from build123d import *

# Parameters (mm, degrees)
CROQUIS6_R              = 7
CROQUIS6_R_2            = 1.4
SALIENTE_EXTRUIR4_DEPTH = 5
REDONDEO2_R             = 3
CROQUIS7_R              = 3
CORTAR_EXTRUIR2_DEPTH   = 3


with BuildPart() as part:
    # Croquis6 → Saliente-Extruir4 (new body)
    with BuildSketch(Plane.ZY.offset(29.169607513)):
        with Locations((65.25, 31.063666838)):
            Circle(CROQUIS6_R)
        with Locations((65.25, 31.063666838)):
            Circle(CROQUIS6_R_2, mode=Mode.SUBTRACT)
    extrude(amount=SALIENTE_EXTRUIR4_DEPTH)

    # Redondeo2
    redondeo2_edges = [part.edges().sort_by_distance(p)[0] for p in [
        (-34.169607513, 31.063666838, 58.25),
    ]]
    fillet(redondeo2_edges, radius=REDONDEO2_R)

    # Croquis7 → Cortar-Extruir2 (cut)
    with BuildSketch(Plane.ZY.offset(34.169607513)):
        with Locations((65.25, 31.063666838)):
            Circle(CROQUIS7_R)
    extrude(amount=-CORTAR_EXTRUIR2_DEPTH, mode=Mode.SUBTRACT)


solid = part.part
Build history of the part. All positions in model axes, mm. A direction names the side the tool comes from. Round coordinates to 2 decimals unless told otherwise and drop trailing zeros. Write each loop counter-clockwise with the first axis right and the second up, starting at its lowest first coordinate (ties: lowest second). Pieces come first, ordered by that corner, then holes. Notation, with made-up numbers: M 89.25,5 L 106.25,5 A32 ccw 106.25,40 Z; hole C 22,89.25 d2. An arc over 180 degrees is marked long. Answer in a Markdown table with one row per item.
1. Flat gauge pins, fed straight in: P1, Ø1.8, axis at y = 30.5, z = 64, coming from the -X side; P2, Ø1, axis at x = -33.5, z = 62, coming from the -Y side; P3, Ø1.5, axis at x = -30.5, z = 63, coming from the +Y side. Where does each tip first touch, or does it go through?
Geometry check:
| item | result |
|---|---|
| P1 | x = -31.17 |
| P2 | y = 25.5 |
| P3 | y = 37.9 |
2. Saw through at C-C (x = -30.1). List the corners of the cut face in (y, z).
Geometry check:
| item | result |
|---|---|
| outline | C 31.06,65.25 d14; hole C 31.06,65.25 d2.8 |
3. Saw through at A-A (z = 65.25). List the corners of the cut face in (x, y).
Geometry check:
| item | result |
|---|---|
| outline | M -34.17,27.06 A3 ccw -31.17,24.06 L -29.17,24.06 L -29.17,29.66 L -31.17,29.66 L -31.17,28.06 L -34.17,28.06 Z; M -34.17,34.06 L -31.17,34.06 L -31.17,32.46 L -29.17,32.46 L -29.17,38.06 L -31.17,38.06 A3 ccw -34.17,35.06 Z |
4. Probe L1, parallel to Y at x = -30.65, z = 65.25; L2, parallel to Y at x = -33.5, z = 62.5; L3, parallel to Z at x = -31.85, y = 29.75. List the from-to ranges inside material, lowest first. Write a range as [from, to].
Geometry check:
| item | result |
|---|---|
| L1 | [24.06, 29.66], [32.46, 38.06] |
| L2 | [25.86, 29.86], [32.26, 36.27] |
| L3 | [58.45, 62.55], [67.95, 72.05] |
5. Which spindle directions (+Z, -Z, +X, -X, +Y, -Y) get a long thin tool onto all of the face, cutting with end or side? Do faces 4 (the face through (-30.156, 31.484, 66.585)), 5 (the face through (-32.69, 33.09, 63.04)). Say none if no direction does.
Geometry check:
| item | result |
|---|---|
| face 4 | +X, -X |
| face 5 | -X |
6. Saw through at B-B (x = -33.3). List the corners of the cut face in (y, z), and give its area (3 significant figures).
Geometry check:
| item | result |
|---|---|
| outline | C 31.06,65.25 d12.22; hole C 31.06,65.25 d6 |
| area | 89.1 mm2 |
7. Mould opens along Y. For faces 1 (the face through (-31.17, 30, 67)), 2 (the face through (-34.17, 34, 67)), 3 (the face through (-30.156, 33.166, 71.927)) say: +Y half, -Y half, draft (parallel to the pull), parting line (faces both ways), or undercut.
Geometry check:
| item | result |
|---|---|
| face 1 | undercut |
| face 2 | draft |
| face 3 | parting line |
